Design review of the part built by this model. Coordinates are the model's own, in mm. A direction names the side the tool comes from. Coordinates: 2 decimals unless noted, no trailing zeros. Loops run counter-clockwise (first coordinate to the right, second up) from the corner with the lowest first, then second, coordinate; pieces in that order, holes last. Notation, with made-up numbers: (-30.75, 37.5) - (-20.75, 37.5) arc R23 cw to (-20.75, 73.5) - close; hole circle Ø9 at (-16, -18). An arc over 180 degrees is marked (long way). Answer in a Markdown table with one row per item. Add a question column.
(1) To check wall thickness, follow L1, parallel to Z at x = 236, y = -1.5; L2, parallel to Z at x = 311.5, y = 44; L3, parallel to Y at x = 213.5, z = -18. State the ranges of each line that lie inside material, in increasing order. Write a range as [from, to].
(2) For faces 1 (the face through (540, 52, 64)), 2 (the face through (331.63, -2.22, 81.97)), list the 3-axis set-ups (+Z, -Z, +X, -X, +Y, -Y) from which the entire face can be reached by the end or side of a thin tool; tool diameter is ignored.
(3) The part is to be moulded in two halves that separate along Y. For faces 3 (the face through (508, 50.3, -65.1)), 4 (the face through (342.27, 84.974, -2.118)), 5 (the face through (347.855, -2.637, -81.958)), say which applies: released by +Y, released by -Y, zero draft, split by the parting line, or undercut.
(4) We need section A-A, the plane x = 213. Write out the cut boundary in (y, z), plus the area to 3 significant figures.
(5) Clearance check with flat-ended pins moving along their axes: pin 1 (3.5 mm diameter, centred on x = 528.5, y = 84, fed in from +Z); pin 2 (7 mm diameter, centred on y = 3, z = 80.5, fed in from +X); pin 3 (6 mm diameter, centred on x = 259, z = -9.5, fed in from -Y); pin 4 (12 mm diameter, centred on x = 451.5, z = 4.5, fed in from +Y). State where each tip first meets the part, or that it passes through.
from build123d import *

# Parameters (mm, degrees)
CUT_EXTRUDE4_REACH              = 555.223
CUT_EXTRUDE1_DEPTH              = 5
BOSS_EXTRUDE1_REACH             = 555.223
SKETCH10_R                      = 2
CIRPATTERN1_COUNT               = 2
CIRPATTERN1_ANGLE               = 80
CIRPATTERN1_THE_OTHER_WAY_COUNT = 2
CIRPATTERN1_THE_OTHER_WAY_ANGLE = 80
F_2_0MM_DOWEL_HOLE1_D           = 2
F_2_0MM_DOWEL_HOLE1_ON_FACE_2_D = 2
F_2_0MM_DOWEL_HOLE1_ON_FACE_3_D = 2
F_2_0MM_DOWEL_HOLE1_ON_FACE_4_D = 2
CUT_EXTRUDE5_START              = -32
CUT_EXTRUDE5_DEPTH              = 32
CIRPATTERN2_COUNT               = 3
CIRPATTERN2_ANGLE               = 136
SKETCH19_R                      = 118.982211047
CUT_EXTRUDE6_DEPTH              = 180


with BuildPart() as part:
    # Sketch1 → Revolve5 (revolve)
    with BuildSketch(Plane.XY, mode=Mode.PRIVATE) as revolve5_sk:
        with BuildLine():
            Line((540, 85), (150, 85))
            add(Edge.make_bspline(
                [(0, 0), (-0.012294225, 3.891554312), (-0.027437579, 8.684958126), (0.361573767, 14.085722357), (0.576098453, 16.090496183), (0.782493435, 17.604822189), (0.986227589, 18.854298664), (1.188670863, 19.931536976), (1.390404268, 20.885679324), (1.591698837, 21.746529091), (1.792703864, 22.533746067), (1.993507167, 23.261083862), (2.253808552, 24.139979457), (2.580573656, 25.146175179), (2.983585386, 26.259501153), (3.385879093, 27.271261727), (3.787683439, 28.201566994), (4.189138614, 29.064817448), (4.590335615, 29.871726974), (5.05331092, 30.74778076), (5.583218589, 31.683457084), (6.185429632, 32.669732492), (6.787226927, 33.590624245), (7.451481511, 34.546094958), (8.182770444, 35.530963646), (8.985083876, 36.540013411), (9.850344603, 37.562485558), (10.782608842, 38.595746542), (11.785011743, 39.636928062), (12.851029789, 40.680352273), (13.983960321, 41.72463117), (15.186170623, 42.768194245), (16.387975322, 43.755294725), (17.654380903, 44.743506811), (18.987602276, 45.731471932), (20.389198856, 46.717890971), (21.790522044, 47.657861765), (23.257103599, 48.59836715), (24.790441056, 49.538186318), (26.391587757, 50.476245251), (28.05829275, 51.412163763), (29.791720393, 52.345056651), (31.59268286, 53.274185034), (33.459445798, 54.199628429), (35.392909821, 55.120726442), (37.459746918, 56.067201212), (39.59327023, 57.006562681), (41.860151348, 57.96659169), (44.193707143, 58.917521836), (46.660609333, 59.885320784), (49.260404933, 60.867669295), (51.99403381, 61.861671206), (54.860992187, 62.865616104), (57.794602823, 63.85555089), (60.861539281, 64.853573463), (64.06149587, 65.858380358), (67.461497598, 66.888166734), (70.995135905, 67.920234745), (74.662088876, 68.953918346), (78.462130407, 69.988575944), (82.462197069, 71.040436012), (86.662284614, 72.107100186), (91.062388571, 73.18640193), (95.662505252, 74.276388609), (100.462631288, 75.375305679), (105.462763855, 76.481579791), (110.662900527, 77.593803027), (116.063039296, 78.710717608), (121.663178505, 79.831201671), (127.529872228, 80.967142806), (133.663251007, 82.116215238), (140.063409966, 83.276352633), (145.198462089, 84.177415336), (148.333178957, 84.715838785), (149.39998937, 84.897876633), (149.733326587, 84.954653305), (149.933332963, 84.98866355), (150, 85)],
                knots=[0, 0, 0, 0, 0.061462209, 0.075705788, 0.085548437, 0.093321935, 0.099856333, 0.105553797, 0.110642995, 0.115267654, 0.119524592, 0.123482434, 0.127191759, 0.134010181, 0.140199136, 0.145901384, 0.151215493, 0.156212588, 0.160945789, 0.165455878, 0.171870938, 0.177937368, 0.183716425, 0.189254732, 0.196326298, 0.203099892, 0.209625632, 0.217492532, 0.225090541, 0.232464167, 0.24106462, 0.249438142, 0.257620809, 0.265641058, 0.274822876, 0.28384341, 0.292725747, 0.301488561, 0.311376345, 0.321146599, 0.330814589, 0.341584449, 0.352255608, 0.362840299, 0.374512001, 0.386101174, 0.398765505, 0.411352526, 0.425006218, 0.438588433, 0.453231339, 0.468927603, 0.484557057, 0.501237456, 0.517857889, 0.535527769, 0.554243231, 0.574001115, 0.593705628, 0.614453399, 0.636242373, 0.65907093, 0.682937829, 0.707842151, 0.733783254, 0.760760729, 0.78877436, 0.81782409, 0.847909993, 0.879032247, 0.912262482, 0.946527454, 0.981827786, 0.994656092, 0.99679374, 0.998931275, 1, 1, 1, 1], degree=3))
            Line((0, 0), (2.999985029, 0))
            Line((2.999985029, 0), (2.999985029, 0.009477573))
            add(Edge.make_bspline(
                [(2.999985029, 0.009477573), (2.993793366, 1.969356524), (2.981962234, 5.911210338), (3.144727077, 11.691517384), (3.670861531, 17.326178467), (4.819198941, 22.729714595), (6.752012755, 27.815986079), (10.434016108, 34.068947754), (16.885973109, 40.769818613), (26.31149284, 47.219276633), (36.588463571, 52.532925143), (47.339293153, 57.041613966), (62.05269101, 62.270744564), (80.889819608, 67.717439736), (103.802651174, 73.170901437), (119.646381092, 76.401254352), (128.250826275, 78.04455103), (129.150186585, 78.215050111), (129.599928532, 78.3)],
                knots=[0, 0, 0, 0, 0.031208253, 0.062416506, 0.093624758, 0.124833011, 0.156041264, 0.187249517, 0.249666023, 0.312082528, 0.374499034, 0.43691554, 0.499332045, 0.624165056, 0.748998068, 0.873333508, 0.88058804, 0.887842573, 0.887842573, 0.887842573, 0.887842573], degree=3))
            add(Edge.make_bspline(
                [(129.599928532, 78.3), (130.04967048, 78.384949889), (130.94927796, 78.554250366), (132.299119739, 78.806440107), (133.649347026, 79.056894297), (134.549738344, 79.222723073), (135, 79.305358628)],
                knots=[0.887842573, 0.887842573, 0.887842573, 0.887842573, 0.895097105, 0.902351638, 0.90960617, 0.916860703, 0.916860703, 0.916860703, 0.916860703], degree=3))
            add(Edge.make_bspline(
                [(135, 79.305358628), (135.450261656, 79.387994183), (140.528235702, 80.316663108), (145.615370758, 81.210683778), (150.253322265, 82)],
                knots=[0.916860703, 0.916860703, 0.916860703, 0.916860703, 0.924115235, 0.99866409, 0.99866409, 0.99866409, 0.99866409], degree=3))
            Line((150.253322265, 82), (540, 82))
            Line((540, 82), (540, 85))
        make_face()
        with BuildLine():
            Line((135, 78.3), (135, 79.305358628))
            add(Edge.make_bspline(
                [(129.599928532, 78.3), (130.04967048, 78.384949889), (130.94927796, 78.554250366), (132.299119739, 78.806440107), (133.649347026, 79.056894297), (134.549738344, 79.222723073), (135, 79.305358628)],
                knots=[0.887842573, 0.887842573, 0.887842573, 0.887842573, 0.895097105, 0.902351638, 0.90960617, 0.916860703, 0.916860703, 0.916860703, 0.916860703], degree=3))
            Line((129.599928532, 78.3), (135, 78.3))
        make_face()
    revolve(revolve5_sk.sketch.rotate(Axis((2.999985029, 0, 0), (1, 0, 0)), 90), axis=Axis((2.999985029, 0, 0), (1, 0, 0)))

    # Cut-Extrude4: up to this face of the body (flat: up to its plane)
    cut_extrude4_end = Plane(part.part.faces().sort_by_distance((135, 0, -78.524309427))[0])
    # Sketch12 → Cut-Extrude4 (cut, up to the picked face)
    with BuildSketch(Plane(origin=(540, 0, 0), x_dir=(0, 0, -1), z_dir=(1, 0, 0)), mode=Mode.PRIVATE) as cut_extrude4_sk1:
        with BuildLine():
            Line((0, 0), (-83.142546062, -17.67249372))
            ThreePointArc((-83.142546062, -17.67249372), (0, -85), (83.142546062, -17.67249372))
            Line((83.142546062, -17.67249372), (0, 0))
        make_face()
    cut_extrude4_tool1 = split(extrude(cut_extrude4_sk1.sketch, amount=-CUT_EXTRUDE4_REACH, mode=Mode.PRIVATE), bisect_by=cut_extrude4_end, keep=Keep.BOTH, mode=Mode.PRIVATE)
    add(cut_extrude4_tool1.solids().sort_by(Axis((540, -40.71553, 0), (-1, 0, 0)))[0], mode=Mode.SUBTRACT)

    # Sketch4 → Cut-Extrude1 (cut)
    with BuildSketch(Plane(origin=(135, 0, 0), x_dir=(0, 0, -1), z_dir=(1, 0, 0))):
        with BuildLine():
            ThreePointArc((40.257565708, -71.845165599), (66.314386739, -48.834429741), (80.55566273, -17.122634693))
            Line((80.55566273, -17.122634693), (77.572346267, -16.488511203))
            Line((77.572346267, -16.488511203), (76.588957137, -16.279485391))
            ThreePointArc((76.588957137, -16.279485391), (64.593537692, -44.255676341), (42.836139649, -65.543536218))
            ThreePointArc((42.836139649, -65.543536218), (41.586655777, -68.710638003), (40.257565708, -71.845165599))
        make_face()
    extrude(amount=-CUT_EXTRUDE1_DEPTH, mode=Mode.SUBTRACT)

    # Sketch10 → Boss-Extrude1 (add, up to next)
    with BuildSketch(Plane(origin=(540, 0, 0), x_dir=(0, 0, -1), z_dir=(1, 0, 0)), mode=Mode.PRIVATE) as boss_extrude1_sk1:
        with Locations((0, 82)):
            Circle(SKETCH10_R)
    boss_extrude1_tool1 = extrude(boss_extrude1_sk1.sketch, amount=-BOSS_EXTRUDE1_REACH, mode=Mode.PRIVATE) - part.part
    boss_extrude1 = boss_extrude1_tool1.solids().sort_by_distance((540, 82, 0))[0]
    add(boss_extrude1)

    # CirPattern1: Boss-Extrude1 ×2 about axis
    cirpattern1_axis = Axis((2.999985029, 0, 0), (-1, 0, 0))
    for i in range(1, CIRPATTERN1_COUNT):
        add(boss_extrude1.rotate(cirpattern1_axis, i * CIRPATTERN1_ANGLE / (CIRPATTERN1_COUNT - 1)))

    # CirPattern1 the other way: Boss-Extrude1 ×2 about axis
    cirpattern1_the_other_way_axis = Axis((2.999985029, 0, 0), (1, 0, 0))
    for i in range(1, CIRPATTERN1_THE_OTHER_WAY_COUNT):
        add(boss_extrude1.rotate(cirpattern1_the_other_way_axis, i * CIRPATTERN1_THE_OTHER_WAY_ANGLE / (CIRPATTERN1_THE_OTHER_WAY_COUNT - 1)))

    # Ø2.0mm Dowel Hole1 (through all)
    with Locations(Plane(origin=(132.5, -78.3, 0), x_dir=(0, 0, 1), z_dir=(0, 1, 0))):
        with Locations((0, 0)):
            Hole(F_2_0MM_DOWEL_HOLE1_D / 2)

    # Ø2.0mm Dowel Hole1 on face 2 (through all)
    with Locations(Plane(origin=(132.5, 0, 78.3), x_dir=(-1, 0, 0), z_dir=(0, 0, -1))):
        with Locations((0, 0)):
            Hole(F_2_0MM_DOWEL_HOLE1_ON_FACE_2_D / 2)

    # Ø2.0mm Dowel Hole1 on face 3 (through all)
    with Locations(Plane(origin=(132.5, 78.3, 0), x_dir=(0, 0, -1), z_dir=(0, -1, 0))):
        with Locations((0, 0)):
            Hole(F_2_0MM_DOWEL_HOLE1_ON_FACE_3_D / 2)

    # Ø2.0mm Dowel Hole1 on face 4 (through all)
    with Locations(Plane(origin=(132.5, 0, -78.3), x_dir=(1, 0, 0), z_dir=(0, 0, 1))):
        with Locations((0, 0)):
            Hole(F_2_0MM_DOWEL_HOLE1_ON_FACE_4_D / 2)

    # Sketch18 → Cut-Extrude5 (cut)
    with BuildSketch(Plane(origin=(540, 0, 0), x_dir=(0, 0, -1), z_dir=(1, 0, 0)).offset(CUT_EXTRUDE5_START)):
        with BuildLine():
            Line((-80.20810326, -17.048758647), (-83.142546062, -17.67249372))
            ThreePointArc((-83.142546062, -17.67249372), (-84.676549338, 7.408238134), (-78.810627638, 31.84156044))
            Line((-78.810627638, 31.84156044), (-76.029076074, 30.71774066))
            Line((-76.029076074, 30.71774066), (0, 0))
            Line((0, 0), (-80.20810326, -17.048758647))
        make_face()
    cut_extrude5 = extrude(amount=CUT_EXTRUDE5_DEPTH, mode=Mode.SUBTRACT)

    # CirPattern2: Cut-Extrude5 ×3 about axis
    cirpattern2_axis = Axis((0, 0, 0), (-1, 0, 0))
    for i in range(1, CIRPATTERN2_COUNT):
        add(cut_extrude5.rotate(cirpattern2_axis, i * CIRPATTERN2_ANGLE / (CIRPATTERN2_COUNT - 1)), mode=Mode.SUBTRACT)

    # Sketch19 → Cut-Extrude6 (cut)
    with BuildSketch(Plane(origin=(135, 0, 0), x_dir=(0, 0, -1), z_dir=(1, 0, 0))):
        Circle(SKETCH19_R)
    extrude(amount=-CUT_EXTRUDE6_DEPTH, mode=Mode.SUBTRACT)


solid = part.part
Responses:
| question | item | result |
|---|---|---|
| 1 | L1 | z = [-84.99, -81.99], [81.99, 84.99] |
| 1 | L2 | z = [-72.73, -69.2], [69.2, 72.73] |
| 1 | L3 | y = [80, 83.07] |
| 2 | face 1 | +Z, -Z, +X, +Y, -Y |
| 2 | face 2 | +X |
| 3 | face 3 | zero draft |
| 3 | face 4 | split by the parting line |
| 3 | face 5 | undercut |
| 4 | outline | (-17.67, -83.14) arc R85 ccw (long way) to (-17.67, 83.14) - (-17.05, 80.21) arc R82 cw to (12.27, 81.08) arc R2 ccw to (16.2, 80.38) arc R82 cw to (81.98, 2) arc R2 ccw to (81.98, -2) arc R82 cw to (16.2, -80.38) arc R2 ccw to (12.27, -81.08) arc R82 cw to (-17.05, -80.21) - close |
| 4 | area | 911 mm2 |
| 5 | pin 1 | stops at z = 0 |
| 5 | pin 2 | stops at x = 508 |
| 5 | pin 3 | stops at y = 81.04 |
| 5 | pin 4 | stops at y = 85 |
